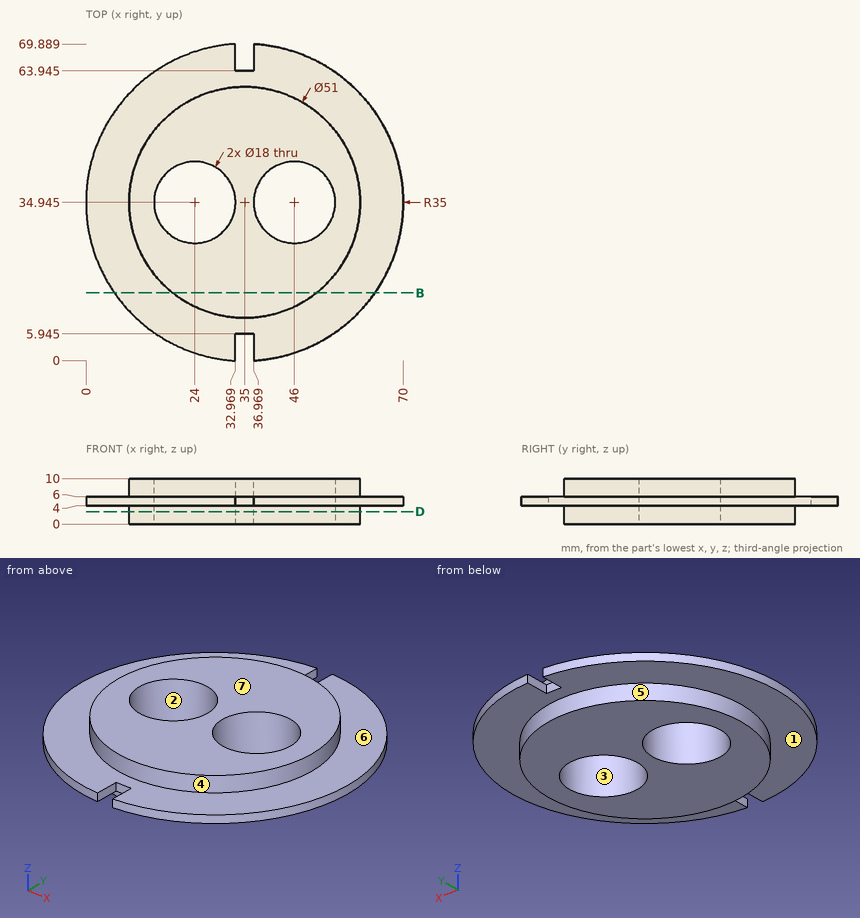
Source: three-view drawing plus pictorial views. Frame: mm from the lowest corner of the part. A direction names the side the tool comes from. Round coordinates to 2 decimals unless told otherwise and drop trailing zeros. Loops run counter-clockwise (first coordinate to the right, second up) from the corner with the lowest first, then second, coordinate; pieces in that order, holes last. Notation, with made-up numbers: (85, -28.5) - (123, -28.5) arc R22 ccw to (123, 0.5) - close; hole circle Ø11 at (81.5, -5.5). An arc over 180 degrees is marked (long way). Write each question's results on one line, items separated by ' | '. Start each with the question number.
1) Access query for the marked faces 5, 6 and 7. Directions: +Z, -Z, +X, -X, +Y, -Y. A direction counts if a zero-diameter tool reaches every point of the face in a straight line with its end or side. Return the directions, or none.
2) First-contact query: P1, Ø2, axis at y = 3, z = 5.5, coming from the +X side (1 decimal); P2, Ø0.6, axis at x = 35.5, z = 5.5, coming from the -Y side (1 decimal); P3, Ø1.6, axis at y = 2, z = 5, coming from the -X side (1 decimal). Flat tips, straight axial feed; report the tip coordinate or a pass-through.
3) Line query: probe 1 along X at (y, z) = (34.5, 2.25); probe 2 along X at (y, z) = (39, 7) (1 decimal); probe 3 along Y at (x, z) = (24, 4.25) (1 decimal). Output: solid intervals per line, ascending. Write a range as [from, to].
4) Cut plane D-D on z = 2.75. Return loops of the section in (x, y) (1 decimal).
5) Cut plane B-B on y = 15. Return loops of the section in (x, z).
6) Mould query, pull axis Y, two halves, no side actions, for the marked faces 1, 2, 3 and 4. Classes: released by +Y, released by -Y, zero draft, split by the parting line, or undercut.
Verdict:
1) face 5: -Z | face 6: +Z | face 7: +Z, +X, -X, +Y, -Y
2) P1: stops at x = 51.4 | P2: stops at y = 5.9 | P3: stops at x = 21.2
3) probe 1: x = [9.5, 15.01], [32.99, 37.01], [54.99, 60.5] | probe 2: x = [9.8, 16], [32, 38], [54, 60.2] | probe 3: y = [1.7, 25.9], [43.9, 68.2]
4) outline: circle Ø51 at (35, 34.9); hole circle Ø18 at (24, 34.9); hole circle Ø18 at (46, 34.9)
5) outline: (6.24, 4) - (19.11, 4) - (19.11, 0) - (50.89, 0) - (50.89, 4) - (63.76, 4) - (63.76, 6) - (50.89, 6) - (50.89, 10) - (19.11, 10) - (19.11, 6) - (6.24, 6) - close
6) face 1: zero draft | face 2: undercut | face 3: undercut | face 4: split by the parting line
